Work out the finished part from the listing and answer in its coordinate system (mm). A direction names the side the tool comes from. Coordinates: 2 decimals unless noted, no trailing zeros. Loops run counter-clockwise (first coordinate to the right, second up) from the corner with the lowest first, then second, coordinate; pieces in that order, holes last. Notation, with made-up numbers: (-19, 88.5) - (10, 88.5) arc R29 ccw to (10, 123.5) - close; hole circle Ø10 at (-25.75, 89). An arc over 180 degrees is marked (long way). Write each question's results on one line, items separated by ' | '. Start each with the question number.
1. Determine the mould class of faces 1 (the flat face through (-39, -7, -46)), 2 (the cylindrical face through (-21.203, 1.521, -16.359)), 3 (the flat face through (50, 2, 1)) for opening direction X: released by +X, released by -X, zero draft, split by the parting line, or undercut.
2. A cutting plane is placed at D-D on y = -3.5. State how many separate pieces and enclosed holes the cut face has, then the cut area to 3 significant figures.
3. A cutting plane is placed at A-A on z = -46.5. Determine the outline of the cut face in (x, y), then the cut area to 3 significant figures.
4. Each of these flat-tipped pins is pushed along its axis until it touches: P1, Ø1, axis at x = -32.5, z = -25.5, coming from the -Y side; P2, Ø5, axis at x = -13.5, z = -3, coming from the +Y side; P3, Ø1.5, axis at y = -4.5, z = 46.5, coming from the -X side. Where does it stop, or does it pass through?
5. Find the intervals of material crossed by line 1 along X through (y, z) = (4, -46.5); line 2 along Y through (x, z) = (46.65, -39); line 3 along X through (y, z) = (1.5, 0), in increasing order. Write a range as [from, to].
6. A cutting plane is placed at B-B on x = -39. Determine the outline of the cut face in (y, z).
7. A cutting plane is placed at C-C on z = 39. Determine the outline of the cut face in (x, y), then the cut area to 3 significant figures.
8. Which of the six approach directions +Z, -Z, +X, -X, +Y, -Y give full straight-line access (tool end or side, diameter ignored) to faces 4 (the flat face through (-43, 5, 47)), 5 (the flat face through (-47, 5, -43)), 6 (the flat face through (-33, 2, -17.5)), 7 (the flat face through (-45, -3, 37)), 8 (the flat face through (-47, -3, 43))?
from build123d import *

# Parameters (mm, degrees)
SKETCH2_W           = 100
SKETCH2_H           = 100
SKETCH2_R           = 12.5
BOSS_EXTRUDE1_DEPTH = 3
SKETCH3_W           = 7
SKETCH3_H           = 7
BOSS_EXTRUDE2_DEPTH = 5
SKETCH4_W           = 3
SKETCH4_H           = 8
SKETCH4_W_2         = 8
SKETCH4_H_2         = 3
BOSS_EXTRUDE3_DEPTH = 7
SKETCH11_R          = 2.5
CUT_EXTRUDE6_DEPTH  = 73.284161474
SKETCH5_R           = 1.6
CUT_EXTRUDE1_DEPTH  = 113.089250154
SKETCH7_R           = 3
CUT_EXTRUDE3_DEPTH  = 10
SKETCH8_R           = 1.6
SKETCH8_R_2         = 1.5
CUT_EXTRUDE4_DEPTH  = 111.308657865
FILLET1_R           = 0.5
CUT_EXTRUDE5_DEPTH  = 10


with BuildPart() as part:
    # Sketch2 → Boss-Extrude1 (new body)
    with BuildSketch(Plane(origin=(0, 0, 0), x_dir=(1, 0, 0), z_dir=(0, 1, 0))):
        Rectangle(SKETCH2_W, SKETCH2_H)
        with Locations(Location((0, 0, 0), (0, 0, 270))):
            Circle(SKETCH2_R, mode=Mode.SUBTRACT)
    extrude(amount=BOSS_EXTRUDE1_DEPTH)

    # Sketch3 → Boss-Extrude2 (add)
    with BuildSketch(Plane(origin=(0, 3, 0), x_dir=(1, 0, 0), z_dir=(0, 1, 0))):
        with Locations((-46.5, 46.5)):
            Rectangle(SKETCH3_W, SKETCH3_H)
        with Locations((46.5, 46.5)):
            Rectangle(SKETCH3_W, SKETCH3_H)
        with Locations((46.5, -46.5)):
            Rectangle(SKETCH3_W, SKETCH3_H)
        with Locations((-46.5, -46.5)):
            Rectangle(SKETCH3_W, SKETCH3_H)
    extrude(amount=BOSS_EXTRUDE2_DEPTH)

    # Sketch4 → Boss-Extrude3 (add)
    with BuildSketch(Plane.XZ):
        with Locations((46.5, -39)):
            Rectangle(SKETCH4_W, SKETCH4_H)
        with Locations((39, 46.5)):
            Rectangle(SKETCH4_W_2, SKETCH4_H_2)
        with Locations((-46.5, 39)):
            Rectangle(SKETCH4_W, SKETCH4_H)
        with Locations((-39, -46.5)):
            Rectangle(SKETCH4_W_2, SKETCH4_H_2)
    extrude(amount=BOSS_EXTRUDE3_DEPTH)

    # Sketch11 → Cut-Extrude6 (cut, through all)
    with BuildSketch(Plane(origin=(0, 8, 0), x_dir=(1, 0, 0), z_dir=(0, 1, 0))):
        with Locations(Location((-46.5, 46.5, 0), (0, 0, 270))):
            Circle(SKETCH11_R)
        with Locations(Location((46.5, 46.5, 0), (0, 0, 270))):
            Circle(SKETCH11_R)
        with Locations(Location((46.5, -46.5, 0), (0, 0, 270))):
            Circle(SKETCH11_R)
        with Locations(Location((-46.5, -46.5, 0), (0, 0, 270))):
            Circle(SKETCH11_R)
    extrude(amount=-CUT_EXTRUDE6_DEPTH, mode=Mode.SUBTRACT)

    # Sketch5 → Cut-Extrude1 (cut, through all)
    with BuildSketch(Plane(origin=(0, 0, 50), x_dir=(-1, 0, 0), z_dir=(0, 0, -1))):
        with Locations(Location((-39, -3.5, 0), (0, 0, 180))):
            Circle(SKETCH5_R)
        with Locations(Location((39, -3.5, 0), (0, 0, 180))):
            Circle(SKETCH5_R)
    extrude(amount=CUT_EXTRUDE1_DEPTH, mode=Mode.SUBTRACT)

    # Sketch7 → Cut-Extrude3 (cut)
    with BuildSketch(Plane.XZ):
        with Locations(Location((30, 0, 0), (0, 0, 270))):
            Circle(SKETCH7_R)
    extrude(amount=-CUT_EXTRUDE3_DEPTH, mode=Mode.SUBTRACT)

    # Sketch8 → Cut-Extrude4 (cut, through all)
    with BuildSketch(Plane(origin=(48, 0, 0), x_dir=(0, 0, -1), z_dir=(1, 0, 0))):
        with Locations((39, -3.5)):
            Circle(SKETCH8_R)
        with Locations(Location((-39, -3.5, 0), (0, 0, 180))):
            Circle(SKETCH8_R_2)
    extrude(amount=-CUT_EXTRUDE4_DEPTH, mode=Mode.SUBTRACT)

    # Fillet1
    fillet1_edges = [part.edges().sort_by_distance(p)[0] for p in [
        (-50, 4, 50),
        (-50, 4, -50),
        (50, 4, -50),
        (50, 4, 50),
    ]]
    fillet(fillet1_edges, radius=FILLET1_R)

    # Sketch9 → Cut-Extrude5 (cut)
    with BuildSketch(Plane(origin=(0, 3, 0), x_dir=(1, 0, 0), z_dir=(0, 1, 0))):
        with BuildLine():
            Line((-41, 17.5), (-24, 17.5))
            ThreePointArc((-24, 17.5), (-21.171572875, 16.328427125), (-20, 13.5))
            Line((-20, 13.5), (-20, -13.5))
            ThreePointArc((-20, -13.5), (-21.171572875, -16.328427125), (-24, -17.5))
            Line((-24, -17.5), (-41, -17.5))
            ThreePointArc((-41, -17.5), (-43.828427125, -16.328427125), (-45, -13.5))
            Line((-45, -13.5), (-45, 13.5))
            ThreePointArc((-45, 13.5), (-43.828427125, 16.328427125), (-41, 17.5))
        make_face()
    extrude(amount=-CUT_EXTRUDE5_DEPTH, mode=Mode.SUBTRACT)


solid = part.part
Values:
1) face 1: zero draft | face 2: undercut | face 3: released by +X
2) separate pieces: 8 | enclosed holes: 0 | area: 58.2 mm^2
3) outline: (-50, 0) - (-49, 0) - (-49, 8) - (-50, 8) - close; (-44, 0) - (-43, 0) - (-43, -7) - (-35, -7) - (-35, 0) - (44, 0) - (44, 8) - (43, 8) - (43, 3) - (-43, 3) - (-43, 8) - (-44, 8) - close; (49, 0) - (50, 0) - (50, 8) - (49, 8) - close; hole circle Ø3.2 at (-39, -3.5) | area: 338 mm^2
4) P1: y = 0 | P2: y = 3 | P3: x = 35
5) line 1: [-50, -49], [-44, -43], [43, 44], [49, 50] | line 2: [-7, -5.1], [-1.9, 3] | line 3: [-50, -45], [-20, -12.5], [12.5, 27], [33, 50]
6) outline: (-7, -48) - (-5.1, -48) - (-5.1, -45) - (-7, -45) - close; (-1.9, -48) - (0, -48) - (0, -50) - (3, -50) - (3, -17.5) - (0, -17.5) - (0, -45) - (-1.9, -45) - close; (0, 17.5) - (3, 17.5) - (3, 50) - (0, 50) - close
7) outline: (-50, 0) - (-48, 0) - (-48, -2) - (-45, -2) - (-45, 0) - (50, 0) - (50, 3) - (-50, 3) - close; (-48, -7) - (-45, -7) - (-45, -5) - (-48, -5) - close | area: 312 mm^2
8) face 4: +Z, -Z, +Y | face 5: +X, -X, +Y | face 6: +Y, -Y | face 7: +Z, -Z, +X, -Y | face 8: +Z, +X, -X, -Y
